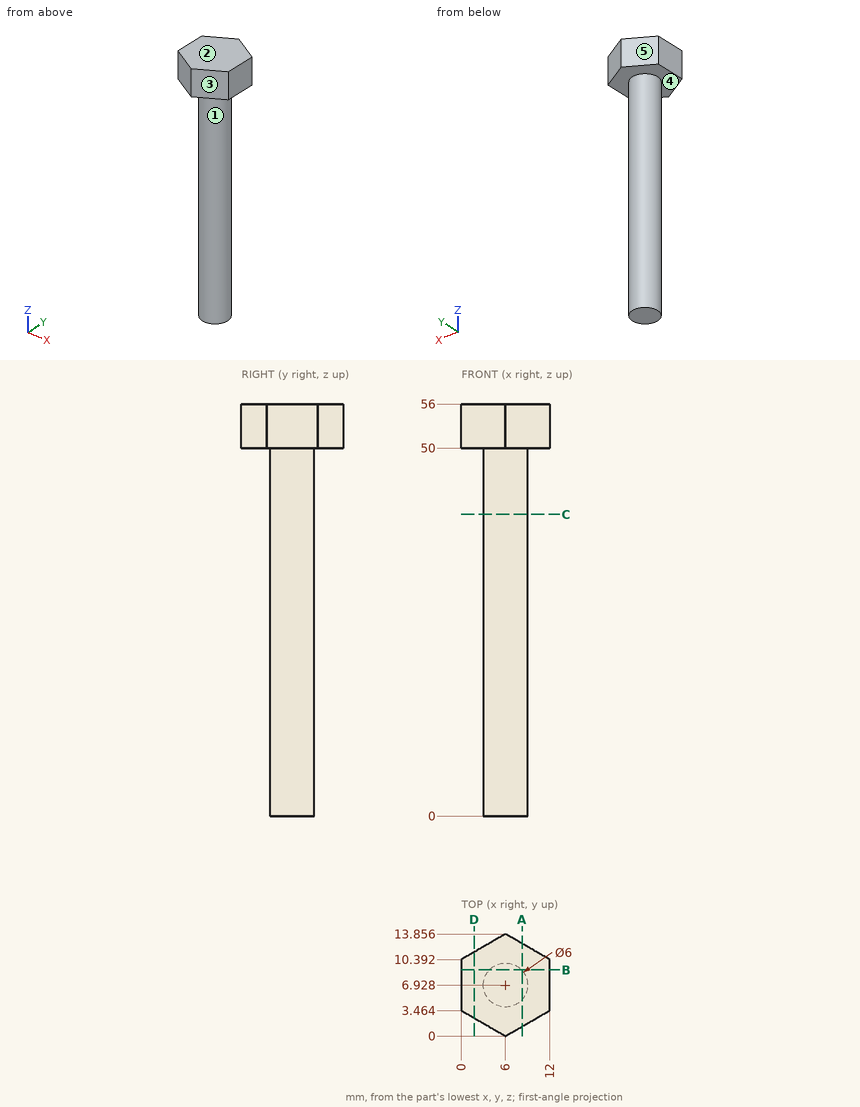
Geometry check sheet. Reference: drawing and pictorial views, mm from the part's lowest x, y, z. A direction names the side the tool comes from. Round coordinates to 2 decimals unless told otherwise and drop trailing zeros. Write each loop counter-clockwise with the first axis right and the second up, starting at its lowest first coordinate (ties: lowest second). Pieces come first, ordered by that corner, then holes. Notation, with made-up numbers: (43.5, 57) -> (67.5, 57) arc R14 ccw to (67.5, 68) -> close; hole circle Ø10 at (-3.5, 66). An arc over 180 degrees is marked (long way). Put each result on its own line as item: value.
1) Release check for a two-part mould opening along X. For the marked faces 3, 4 and 5 record: pulls with the +X half, pulls with the -X half, needs draft (parallel to the pull), parting line crosses it, or undercut.
Recorded:
face 3: pulls with the +X half
face 4: needs draft
face 5: pulls with the -X half
2) Depth check by flat-ended pin: P1, Ø6, axis at y = 10, z = 16, coming from the -X side; P2, Ø1, axis at x = 10, z = 39, coming from the -Y side; P3, Ø3, axis at y = 11, z = 41.5, coming from the +X side (1 decimal); P4, Ø3.5, axis at x = 3.5, y = 9, coming from the -Z side. Enter the tip coordinate at first touch or a pass-through.
Recorded:
P1: stops at x = 3
P2: passes through
P3: stops at x = 7.5
P4: stops at z = 0
3) Cross-section at A-A, the plane x = 8.25. Enter the section's corners in (y, z), plus the area to 3 significant figures.
Recorded:
outline: (1.3, 50) -> (4.94, 50) -> (4.94, 0) -> (8.91, 0) -> (8.91, 50) -> (12.56, 50) -> (12.56, 56) -> (1.3, 56) -> close
area: 266 mm2
4) Cross-section at D-D, the plane x = 1.75. Enter the section's corners in (y, z).
Recorded:
outline: (2.45, 50) -> (11.4, 50) -> (11.4, 56) -> (2.45, 56) -> close
5) Cross-section at B-B, the plane y = 9. Enter the section's corners in (x, z), plus the area to 3 significant figures.
Recorded:
outline: (0, 50) -> (3.83, 50) -> (3.83, 0) -> (8.17, 0) -> (8.17, 50) -> (12, 50) -> (12, 56) -> (0, 56) -> close
area: 289 mm2
6) Cross-section at C-C, the plane z = 41. Enter the section's corners in (x, y).
Recorded:
outline: circle Ø6 at (6, 6.93)
7) Access from +Z, -Z, +X, -X, +Y, -Y to the whole of each face (thin tool, end or side, straight path). Record for the marked faces 1 and 2.
Recorded:
face 1: -Z
face 2: +Z, +X, -X, +Y, -Y
8) Thickness scan on probe 1 along Z at (x, y) = (8.75, 2.25); probe 2 along X at (y, z) = (7, 39); probe 3 along Y at (x, z) = (4, 7.5) (1 decimal). Record the ranges inside material, lowest first. Write a range as from..to.
Recorded:
probe 1: z = 50..56
probe 2: x = 3..9
probe 3: y = 4.7..9.2
